Build history of the part. All positions in model axes, mm. Round coordinates to 2 decimals unless told otherwise and drop trailing zeros. Write each loop counter-clockwise with the first axis right and the second up, starting at its lowest first coordinate (ties: lowest second). Pieces come first, ordered by that corner, then holes. Notation, with made-up numbers: (23.5, 85) -> (79.5, 85) arc R23 cw to (79.5, 108) -> close; hole circle Ø1 at (57, 15). An arc over 180 degrees is marked (long way). Answer as CSV lines item,"result".
from build123d import *

# Parameters (mm, degrees)
F0_R     = 1.75
F1_DEPTH = 3
F2_DEPTH = 200
F3_R     = 1.75
F4_DEPTH = 3


with BuildPart() as f1:
    # F0 (on Right) → F1 (new body)
    with BuildSketch(Plane.YZ):
        Polygon((-3, 2.5), (-10, 2.5), (-10, 5.5), (-15.5, 2.03124969), (-15.5, -1.96875031), (-10, -5.5), (-10, -2.5), (-3, -2.5), align=None)
        with Locations((-11.75, 0)):
            Circle(F0_R, mode=Mode.SUBTRACT)
    extrude(amount=F1_DEPTH)



with BuildPart() as f1b:
    # F0 (on Right) → F1, piece 2 (new body)
    with BuildSketch(Plane.YZ):
        Polygon((15.5, 2.03124969), (10, 5.5), (10, 2.5), (3, 2.5), (3, -2.5), (10, -2.5), (10, -5.5), (15.5, -1.96875031), align=None)
        with Locations((11.75, 0)):
            Circle(F0_R, mode=Mode.SUBTRACT)
    extrude(amount=F1_DEPTH)


with BuildPart() as f1_1:
    add(f1.part)

    add(f1b.part)  # F2 merges F1b
    # F0 (on Right) → F2 (join)
    with BuildSketch(Plane.YZ):
        Polygon((-10, 5.5), (-10, 2.5), (-3, 2.5), (-3, -2.5), (-10, -2.5), (-10, -5.5), (10, -5.5), (10, -2.5), (3, -2.5), (3, 2.5), (10, 2.5), (10, 5.5), align=None)
    extrude(amount=F2_DEPTH)

    # F3 (on face) → F4 (join)
    with BuildSketch(Plane.YZ.offset(200)):
        Polygon((-3, 2.5), (-10, 2.5), (-10, 5.5), (-15.5, 2.03124969), (-15.5, -1.96875031), (-10, -5.5), (-10, -2.5), (-3, -2.5), align=None)
        with Locations((-11.75, 0)):
            Circle(F3_R, mode=Mode.SUBTRACT)
        Polygon((15.5, 2.03124969), (10, 5.5), (10, 2.5), (3, 2.5), (3, -2.5), (10, -2.5), (10, -5.5), (15.5, -1.96875031), align=None)
        with Locations((11.75, 0)):
            Circle(F3_R, mode=Mode.SUBTRACT)
    extrude(amount=-F4_DEPTH)


solid = f1_1.part
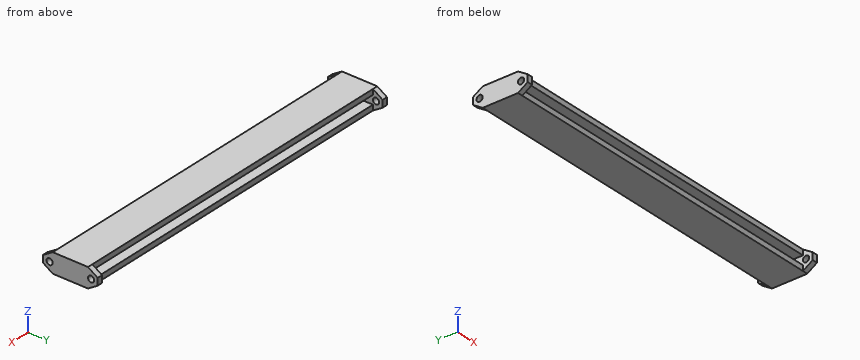
1. Probe line 1 along X through (y, z) = (9.5, -1.75); line 2 along Z through (x, y) = (113, -9); line 3 along Y through (x, z) = (174, 3.25). List the from-to ranges inside material, lowest first.
Results found:
line 1,"x = 0 to 3, 197 to 200"
line 2,"z = -5.5 to -2.5, 2.5 to 5.5"
line 3,"y = -10 to 10"
2. Cut at A-A, the plane x = 58. Write the cut outline in (y, z).
Results found:
outline,"(-10, -5.5) -> (10, -5.5) -> (10, -2.5) -> (3, -2.5) -> (3, 2.5) -> (10, 2.5) -> (10, 5.5) -> (-10, 5.5) -> (-10, 2.5) -> (-3, 2.5) -> (-3, -2.5) -> (-10, -2.5) -> close"
3. Cut at B-B, the plane y = 7. Write the cut outline in (x, z), then the cut area to 3 significant figures.
Results found:
outline,"(0, -5.5) -> (200, -5.5) -> (200, 5.5) -> (0, 5.5) -> close; hole (3, -2.5) -> (197, -2.5) -> (197, 2.5) -> (3, 2.5) -> close"
area,"1,230 mm2"
4. Cut at C-C, the plane z = 0. Write the cut outline in (x, y).
Results found:
outline,"(0, -15.5) -> (3, -15.5) -> (3, -13.5) -> (0, -13.5) -> close; (0, -10) -> (3, -10) -> (3, -3) -> (197, -3) -> (197, -10) -> (200, -10) -> (200, 10) -> (197, 10) -> (197, 3) -> (3, 3) -> (3, 10) -> (0, 10) -> close; (0, 13.5) -> (3, 13.5) -> (3, 15.5) -> (0, 15.5) -> close; (197, -15.5) -> (200, -15.5) -> (200, -13.5) -> (197, -13.5) -> close; (197, 13.5) -> (200, 13.5) -> (200, 15.5) -> (197, 15.5) -> close"
5. Drop flat-ended pins along their axis: pin 1 Ø6 at (y, z) = (6, -2.5) entering from -X; pin 2 Ø3.5 at (x, z) = (101, 4.5) entering from +Y; pin 3 Ø4 at (x, z) = (154.5, -1.5) entering from -Y; pin 4 Ø1.5 at (x, z) = (51.5, -1) entering from +Y. Give the stop position or say it passes through.
Results found:
pin 1,"stops at x = 0"
pin 2,"stops at y = 10"
pin 3,"stops at y = -10"
pin 4,"stops at y = 3"
6. Cut at D-D, the plane y = -11.75. Write the cut outline in (x, z), then the cut area to 3 significant figures.
Results found:
outline,"(0, -4.38) -> (3, -4.38) -> (3, -1.75) -> (0, -1.75) -> close; (0, 1.75) -> (3, 1.75) -> (3, 4.4) -> (0, 4.4) -> close; (197, -4.38) -> (200, -4.38) -> (200, -1.75) -> (197, -1.75) -> close; (197, 1.75) -> (200, 1.75) -> (200, 4.4) -> (197, 4.4) -> close"
area,"31.6 mm2"
